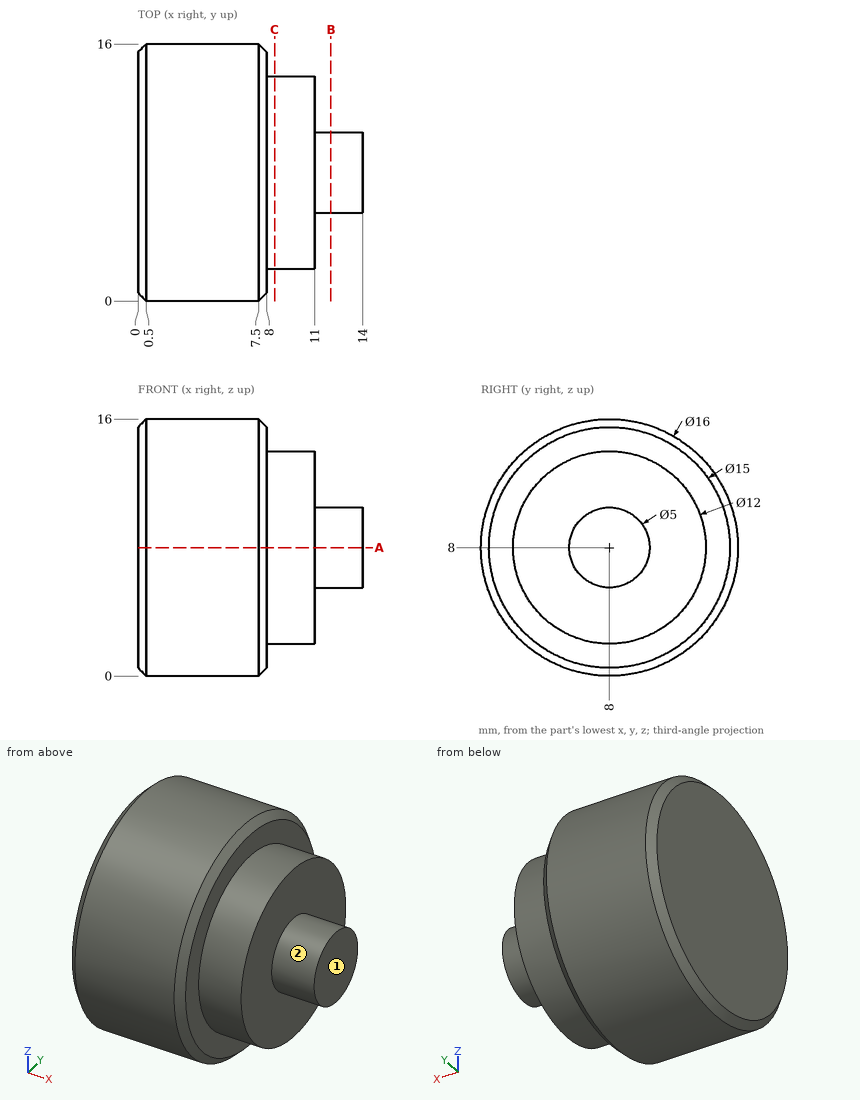
Source: three-view drawing plus pictorial views. Frame: mm from the lowest corner of the part. A direction names the side the tool comes from. Give positions to 0.01 mm unless a question says otherwise; leave off trailing zeros. Loops run counter-clockwise (first coordinate to the right, second up) from the corner with the lowest first, then second, coordinate; pieces in that order, holes last. Notation, with made-up numbers: (68, 26.25) -> (102, 26.25) arc R6 cw to (102, 37.25) -> close; hole circle Ø4 at (46.5, 84). An arc over 180 degrees is marked (long way). Use a Markdown table: item, result. Add a question column.
(1) First-contact query: pin 1 Ø4 at (x, y) = (9.5, 5.5) entering from -Z; pin 2 Ø4 at (x, y) = (8, 13) entering from +Z; pin 3 Ø1 at (y, z) = (3, 2.5) entering from +X. Flat tips, straight axial feed; report the tip coordinate or a pass-through.
(2) Section query A-A (z = 8). Output: boundary loops of the cut face in (x, y).
(3) Ray query, line 1 (X direction, y = 3, z = 8); line 2 (X direction, y = 2.5, z = 5.25); line 3 (Y direction, x = 1.25, z = 7.75). Return the intervals inside material, ascending.
(4) Access query for the marked faces 1 and 2. Directions: +Z, -Z, +X, -X, +Y, -Y. A direction counts if a zero-diameter tool reaches every point of the face in a straight line with its end or side. Return the directions, or none.
(5) Section query B-B (x = 12). Output: boundary loops of the cut face in (y, z), then the cut area to 3 significant figures.
(6) Section query C-C (x = 8.5). Output: boundary loops of the cut face in (y, z).
Checked values:
| question | item | result |
|---|---|---|
| 1 | pin 1 | z = 0.32 |
| 1 | pin 2 | z = 15.39 |
| 1 | pin 3 | x = 8 |
| 2 | outline | (0, 0.5) -> (0.5, 0) -> (7.5, 0) -> (8, 0.5) -> (8, 2) -> (11, 2) -> (11, 5.5) -> (14, 5.5) -> (14, 10.5) -> (11, 10.5) -> (11, 14) -> (8, 14) -> (8, 15.5) -> (7.5, 16) -> (0.5, 16) -> (0, 15.5) -> close |
| 3 | line 1 | 0 to 11 |
| 3 | line 2 | 0 to 8 |
| 3 | line 3 | 0 to 16 |
| 4 | face 1 | +Z, -Z, +X, +Y, -Y |
| 4 | face 2 | +X |
| 5 | outline | circle Ø5 at (8, 8) |
| 5 | area | 19.6 mm^2 |
| 6 | outline | circle Ø12 at (8, 8) |
